Here's the drawing with two shaded views (mm, measured from the low corner). I have some questions. A direction names the side the tool comes from. Coordinates: 2 decimals unless noted, no trailing zeros. Write each loop counter-clockwise with the first axis right and the second up, starting at its lowest first coordinate (ties: lowest second). Pieces come first, ordered by that corner, then holes.
Item 1: Thinking about a two-plate mould opening in X: for the marked faces 1, 2 and 3, which applies, +X half, -X half, draft (parallel to the pull), parting line (faces both ways), or undercut?
Item 2: I want a section at D-D on y = 2. Please give me the cut outline in (x, z), then the cut area to 3 significant figures.
Item 3: If I drill on probe 1 along Y at (x, z) = (16, 1.2); probe 2 along Z at (x, y) = (6, 28.5); probe 3 along Y at (x, z) = (21, 8), over which ranges is the centre line in solid material (lowest first)?
Item 4: I want a section at A-A on x = 4.5. Please give me the cut outline in (y, z), then the cut area to 3 significant figures.
Item 5: I want a section at B-B on y = 20.5. Please give me the cut outline in (x, z), then the cut area to 3 significant figures.
Item 6: Which directions (+Z, -Z, +X, -X, +Y, -Y) give clear straight access to the entire face, cutting with the end or side of a thin tool? Please do the marked faces 4, 5 and 6.
Item 7: I want a section at C-C on x = 16. Please give me the cut outline in (y, z), then the cut area to 3 significant figures.
Item 8: For P1, Ø5, axis at y = 17.5, z = 34.5, coming from the -X side; P2, Ø14, axis at x = 12, y = 20, coming from the -Z side, each with a flat end and sliding along its axis, tell me the tip position at first contact or that it passes through.
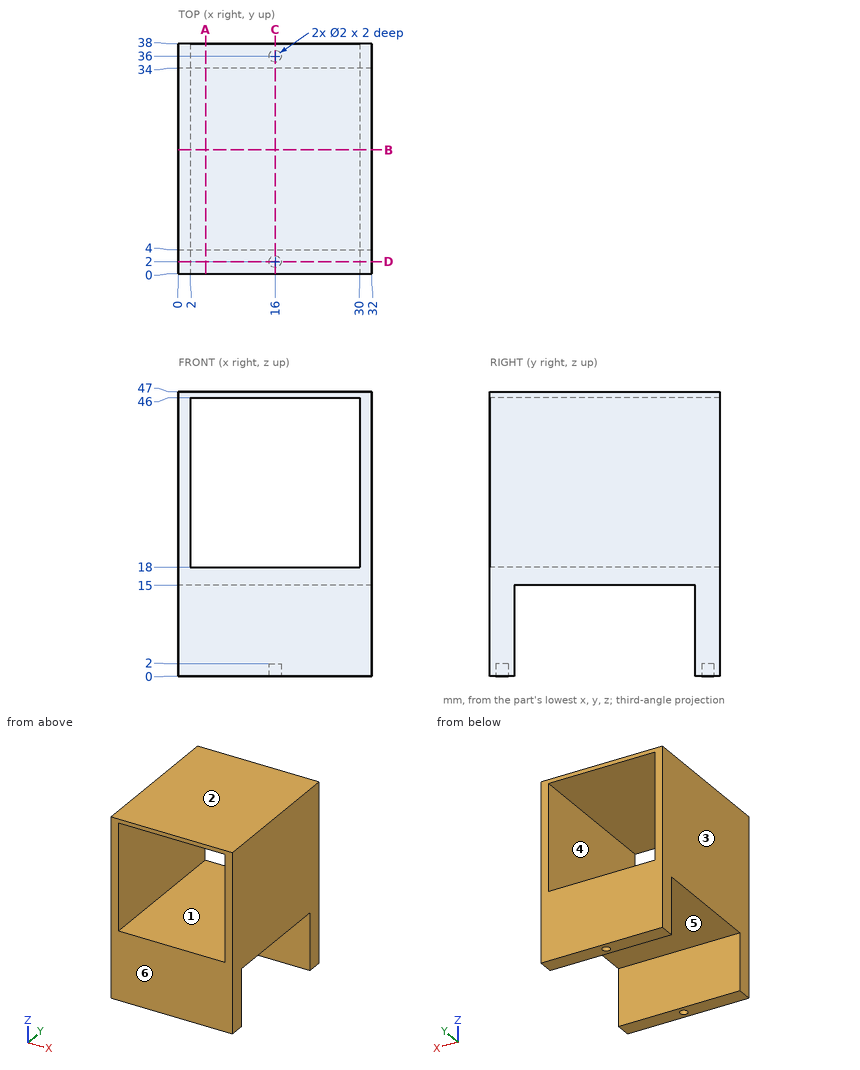
Response values:
1. face 1: undercut
1. face 2: draft
1. face 3: -X half
2. outline: (0, 0) - (15, 0) - (15, 2) - (17, 2) - (17, 0) - (32, 0) - (32, 47) - (0, 47) - close; hole (2, 18) - (30, 18) - (30, 46) - (2, 46) - close
2. area: 716 mm2
3. probe 1: y = 0 to 1, 3 to 4, 34 to 35, 37 to 38
3. probe 2: z = 15 to 18, 46 to 47
3. probe 3: y = 0 to 4, 34 to 38
4. outline: (0, 0) - (4, 0) - (4, 15) - (34, 15) - (34, 0) - (38, 0) - (38, 18) - (0, 18) - close; (0, 46) - (38, 46) - (38, 47) - (0, 47) - close
4. area: 272 mm2
5. outline: (0, 15) - (32, 15) - (32, 47) - (0, 47) - close; hole (2, 18) - (30, 18) - (30, 46) - (2, 46) - close
5. area: 240 mm2
6. face 4: +Y, -Y
6. face 5: -Z, +X, -X
6. face 6: +Z, -Z, +X, -X, -Y
7. outline: (0, 0) - (1, 0) - (1, 2) - (3, 2) - (3, 0) - (4, 0) - (4, 15) - (34, 15) - (34, 0) - (35, 0) - (35, 2) - (37, 2) - (37, 0) - (38, 0) - (38, 18) - (0, 18) - close; (0, 46) - (38, 46) - (38, 47) - (0, 47) - close
7. area: 264 mm2
8. P1: stops at x = 0
8. P2: stops at z = 15
